Answer from the drawing. Dimensions are ordinates in mm from the lowest x, y and z of the part. A direction names the side the tool comes from. Coordinates: 2 decimals unless noted, no trailing zeros. Write each loop counter-clockwise with the first axis right and the second up, starting at its lowest first coordinate (ties: lowest second). Pieces come first, ordered by that corner, then holes. Notation, with made-up numbers: (25.5, -14) - (63.5, -14) arc R7 cw to (63.5, -4) - close; hole circle Ø9 at (50.5, 9.5). An arc over 180 degrees is marked (long way). Return JSON: item names as keys, results as strings.
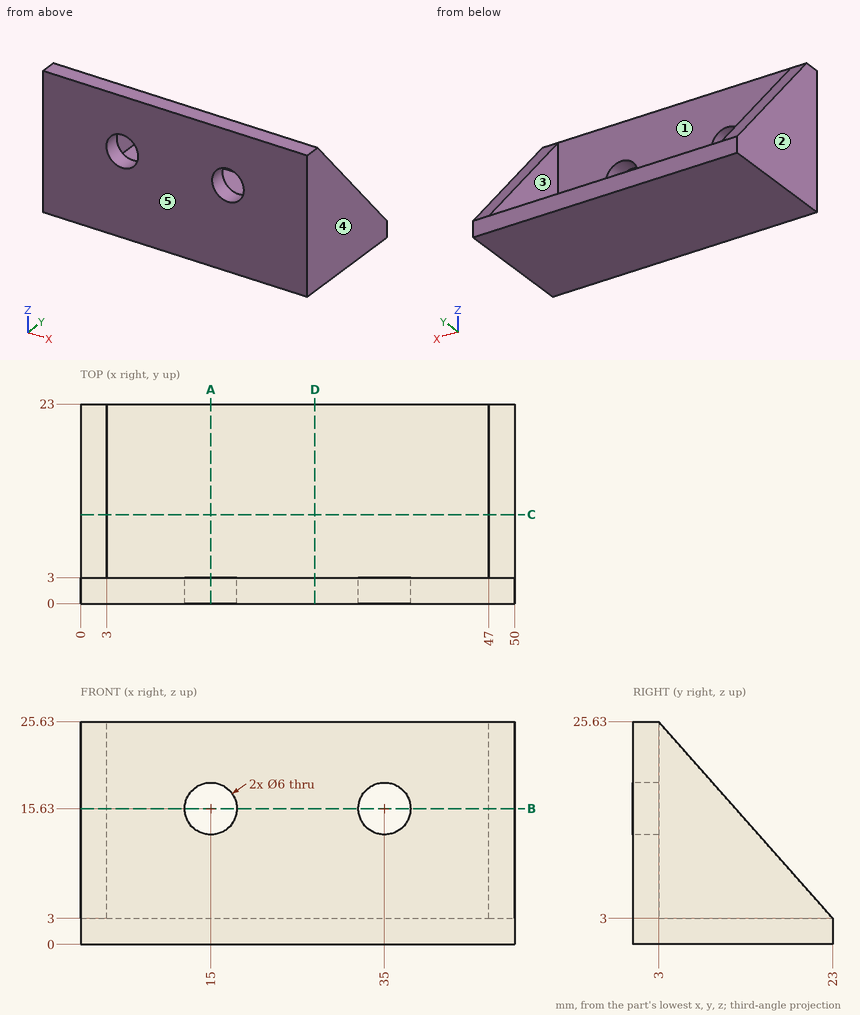
(1) A cutting plane is placed at A-A (x = 15). Determine the outline of the cut face in (y, z), and give its area (3 significant figures).
Answer:
{"outline": "(0, 0) - (23, 0) - (23, 3) - (3, 3) - (3, 12.63) - (0, 12.63) - close; (0, 18.63) - (3, 18.63) - (3, 25.63) - (0, 25.63) - close", "area": "119 mm²"}
(2) A cutting plane is placed at B-B (z = 15.63). Determine the outline of the cut face in (x, y), and give its area (3 significant figures).
Answer:
{"outline": "(0, 0) - (12, 0) - (12, 3) - (3, 3) - (3, 11.84) - (0, 11.84) - close; (18, 0) - (32, 0) - (32, 3) - (18, 3) - close; (38, 0) - (50, 0) - (50, 11.84) - (47, 11.84) - (47, 3) - (38, 3) - close", "area": "167 mm²"}
(3) A cutting plane is placed at C-C (y = 10.25). Determine the outline of the cut face in (x, z).
Answer:
{"outline": "(0, 0) - (50, 0) - (50, 17.43) - (47, 17.43) - (47, 3) - (3, 3) - (3, 17.43) - (0, 17.43) - close"}
(4) Determine the mould class of the marked faces 3, 4 and 5 for opening direction X: +X half, -X half, draft (parallel to the pull), parting line (faces both ways), or undercut.
Answer:
{"face 3": "undercut", "face 4": "+X half", "face 5": "draft"}
(5) Flat-ended cylindrical pins translate along their axes: P1, Ø10, axis at x = 22, y = 17, coming from the +Z side; P2, Ø1, axis at x = 37.5, z = 19, coming from the +Y side. Find the tip coordinate at first contact, or state that the pin passes through.
Answer:
{"P1": "z = 3", "P2": "y = 3"}
(6) Which of the six approach directions +Z, -Z, +X, -X, +Y, -Y give full straight-line access (tool end or side, diameter ignored) to the marked faces 1 and 2?
Answer:
{"face 1": "+Z, +Y", "face 2": "+Z, -Z, -X, +Y, -Y"}
(7) A cutting plane is placed at D-D (x = 27). Determine the outline of the cut face in (y, z), and give its area (3 significant figures).
Answer:
{"outline": "(0, 0) - (23, 0) - (23, 3) - (3, 3) - (3, 25.63) - (0, 25.63) - close", "area": "137 mm²"}
(8) Straight lines are drawn through the part: line 1 (X direction, y = 1.7, z = 15.63); line 2 (X direction, y = 4.5, z = 5); line 3 (Z direction, x = 35, y = 1.7). For each, find the intervals that lie inside material, in ascending order. Write a range as from..to.
Answer:
{"line 1": "0..12, 18..32, 38..50", "line 2": "0..3, 47..50", "line 3": "0..12.63, 18.63..25.63"}
